from build123d import *

# Parameters (mm, degrees)
SKETCH1_W           = 13.2
SKETCH1_H           = 12.5
BOSS_EXTRUDE1_DEPTH = 6
SKETCH2_R           = 3.4
BOSS_EXTRUDE2_DEPTH = 6.5
BOSS_EXTRUDE3_DEPTH = 5


with BuildPart() as part:
    # Sketch1 → Boss-Extrude1 (new body)
    with BuildSketch(Plane(origin=(0, 0, 0), x_dir=(1, 0, 0), z_dir=(0, 1, 0))):
        Rectangle(SKETCH1_W, SKETCH1_H)
    extrude(amount=BOSS_EXTRUDE1_DEPTH)

    # Sketch2 → Boss-Extrude2 (add)
    with BuildSketch(Plane(origin=(0, 6, 0), x_dir=(1, 0, 0), z_dir=(0, 1, 0))):
        Circle(SKETCH2_R)
    extrude(amount=BOSS_EXTRUDE2_DEPTH)

    # Sketch3 → Boss-Extrude3 (add)
    with BuildSketch(Plane(origin=(0, 12.5, 0), x_dir=(1, 0, 0), z_dir=(0, 1, 0))):
        with BuildLine():
            Line((-1.5, -2.598076211), (-1.5, 2.598076211))
            ThreePointArc((-1.5, 2.598076211), (3, 0), (-1.5, -2.598076211))
        make_face()
    extrude(amount=BOSS_EXTRUDE3_DEPTH)


solid = part.part
Here's how the part is built. I have some questions about the finished solid (model axes, mm). A direction names the side the tool comes from. Coordinates: 2 decimals unless noted, no trailing zeros. Order: outer loops, then holes, each group sorted by start corner. A loop starts at its lowest first (then second) coordinate and runs counter-clockwise, first axis right, second up.
Item 1: If we section it at A-A on x = 0: List the corners of the cut face in (y, z) for me.
Result sheet:
outline: (0, -6.25) - (6, -6.25) - (6, -3.4) - (12.5, -3.4) - (12.5, -3) - (17.5, -3) - (17.5, 3) - (12.5, 3) - (12.5, 3.4) - (6, 3.4) - (6, 6.25) - (0, 6.25) - close
Item 2: If we section it at C-C on y = 8: List the corners of the cut face in (x, z) for me, plus the area to 3 significant figures.
Result sheet:
outline: circle Ø6.8 at (0, 0)
area: 36.3 mm2
Item 3: I need wall thicknesses on line 1 (Z direction, x = 0, y = 7.5); line 2 (Y direction, x = -4, z = 5.75); line 3 (Y direction, x = -2.75, z = 1). Which ranges of each line are inside material? Lowest first, please.
Result sheet:
line 1: z = -3.4 to 3.4
line 2: y = 0 to 6
line 3: y = 0 to 12.5
Item 4: If we section it at B-B on z = 0: List the corners of the cut face in (x, y) for me, plus the area to 3 significant figures.
Result sheet:
outline: (-6.6, 0) - (6.6, 0) - (6.6, 6) - (3.4, 6) - (3.4, 12.5) - (3, 12.5) - (3, 17.5) - (-1.5, 17.5) - (-1.5, 12.5) - (-3.4, 12.5) - (-3.4, 6) - (-6.6, 6) - close
area: 146 mm2
Item 5: For faces 1 (the face through (-0.74, 9.2, 3.32)), 2 (the face through (6.6, 3, 0)), 3 (the face through (-1.5, 15, 0)), which set-ups out of +Z, -Z, +X, -X, +Y, -Y let a thin tool reach every point of the face, with its end or its side?
Result sheet:
face 1: +Y
face 2: +Z, -Z, +X, +Y, -Y
face 3: +Z, -Z, -X, +Y
Item 6: If we section it at D-D on z = -4.75: List the corners of the cut face in (x, y) for me, plus the area to 3 significant figures.
Result sheet:
outline: (-6.6, 0) - (6.6, 0) - (6.6, 6) - (-6.6, 6) - close
area: 79.2 mm2
Item 7: For P1, Ø2, axis at y = 7.5, z = -1.5, coming from the +X side; P2, Ø1.5, axis at y = 8, z = 3, coming from the -X side; P3, Ø2.5, axis at y = 14.5, z = 0.5, coming from the -X side, each with a flat end and sliding along its axis, tell me the tip position at first contact or that it passes through.
Result sheet:
P1: stops at x = 3.36
P2: stops at x = -2.55
P3: stops at x = -1.5
